from build123d import *

# Parameters (mm, degrees)
SKETCH1_R           = 1.65
BOSS_EXTRUDE1_DEPTH = 3
BOSS_EXTRUDE2_START = -3
BOSS_EXTRUDE2_DEPTH = 3
SKETCH3_R           = 1.35
CUT_EXTRUDE1_DEPTH  = 3
BOSS_EXTRUDE3_START = 2
SKETCH4_R           = 2.85
SKETCH4_R_2         = 1.35
BOSS_EXTRUDE3_DEPTH = 2


with BuildPart() as part:
    # Sketch1 → Boss-Extrude1 (new body)
    with BuildSketch(Plane(origin=(0, 0, 0), x_dir=(1, 0, 0), z_dir=(0, 1, 0))):
        with BuildLine():
            Line((-91, 63), (-11.779218989, 63))
            ThreePointArc((-11.779218989, 63), (-9.093788212, 62.217636961), (-7.248750147, 60.115384615))
            ThreePointArc((-7.248750147, 60.115384615), (0, 55.5), (7.248750147, 60.115384615))
            ThreePointArc((7.248750147, 60.115384615), (9.093788212, 62.217636961), (11.779218989, 63))
            Line((11.779218989, 63), (91, 63))
            ThreePointArc((91, 63), (94.535533906, 61.535533906), (96, 58))
            Line((96, 58), (96, -58))
            ThreePointArc((96, -58), (94.535533906, -61.535533906), (91, -63))
            Line((91, -63), (11.779218989, -63))
            ThreePointArc((11.779218989, -63), (9.093788212, -62.217636961), (7.248750147, -60.115384615))
            ThreePointArc((7.248750147, -60.115384615), (0, -55.5), (-7.248750147, -60.115384615))
            ThreePointArc((-7.248750147, -60.115384615), (-9.093788212, -62.217636961), (-11.779218989, -63))
            Line((-11.779218989, -63), (-91, -63))
            ThreePointArc((-91, -63), (-94.535533906, -61.535533906), (-96, -58))
            Line((-96, -58), (-96, 58))
            ThreePointArc((-96, 58), (-94.535533906, 61.535533906), (-91, 63))
        make_face()
        with Locations(Location((-91, 58, 0), (0, 0, 270))):
            Circle(SKETCH1_R, mode=Mode.SUBTRACT)
        with Locations(Location((91, 58, 0), (0, 0, 270))):
            Circle(SKETCH1_R, mode=Mode.SUBTRACT)
        with Locations(Location((91, -58, 0), (0, 0, 270))):
            Circle(SKETCH1_R, mode=Mode.SUBTRACT)
        with Locations(Location((-91, -58, 0), (0, 0, 270))):
            Circle(SKETCH1_R, mode=Mode.SUBTRACT)
        with BuildLine():
            Line((-81, 53), (-15, 53))
            ThreePointArc((-15, 53), (-7.928932188, 50.071067812), (-5, 43))
            Line((-5, 43), (-5, -43))
            ThreePointArc((-5, -43), (-7.928932188, -50.071067812), (-15, -53))
            Line((-15, -53), (-81, -53))
            ThreePointArc((-81, -53), (-84.535533906, -51.535533906), (-86, -48))
            Line((-86, -48), (-86, 48))
            ThreePointArc((-86, 48), (-84.535533906, 51.535533906), (-81, 53))
        make_face(mode=Mode.SUBTRACT)
        with BuildLine():
            Line((86, -48), (86, 48))
            ThreePointArc((86, 48), (84.535533906, 51.535533906), (81, 53))
            Line((81, 53), (15, 53))
            ThreePointArc((15, 53), (7.928932188, 50.071067812), (5, 43))
            Line((5, 43), (5, -43))
            ThreePointArc((5, -43), (7.928932188, -50.071067812), (15, -53))
            Line((15, -53), (81, -53))
            ThreePointArc((81, -53), (84.535533906, -51.535533906), (86, -48))
        make_face(mode=Mode.SUBTRACT)
    extrude(amount=BOSS_EXTRUDE1_DEPTH)

    # Sketch2 → Boss-Extrude2 (add)
    with BuildSketch(Plane(origin=(0, 3, 0), x_dir=(1, 0, 0), z_dir=(0, 1, 0)).offset(BOSS_EXTRUDE2_START)):
        with BuildLine():
            Line((-42, -39.5), (-86, -39.5))
            Line((-86, -39.5), (-86, -48))
            ThreePointArc((-86, -48), (-85.942088629, -48.758788496), (-85.769696007, -49.5))
            Line((-85.769696007, -49.5), (-42, -49.5))
            Line((-42, -49.5), (-7.400657923, -49.5))
            ThreePointArc((-7.400657923, -49.5), (-5.619343819, -46.464576398), (-5, -43))
            Line((-5, -43), (-5, -39.5))
            Line((-5, -39.5), (-42, -39.5))
        make_face()
        Polygon((-86, 18.5), (-86, 8.5), (-42, 8.5), (-5, 8.5), (-5, 18.5), (-42, 18.5), align=None)
    extrude(amount=BOSS_EXTRUDE2_DEPTH)

    # Sketch3 → Cut-Extrude1 (cut)
    with BuildSketch(Plane(origin=(0, 3, 0), x_dir=(1, 0, 0), z_dir=(0, 1, 0))):
        with Locations(Location((-42, -44.5, 0), (0, 0, 270))):
            Circle(SKETCH3_R)
        with Locations(Location((-91, -44.5, 0), (0, 0, 270))):
            Circle(SKETCH3_R)
        with Locations(Location((-42, 13.5, 0), (0, 0, 270))):
            Circle(SKETCH3_R)
        with Locations(Location((-91, 13.5, 0), (0, 0, 270))):
            Circle(SKETCH3_R)
    extrude(amount=-CUT_EXTRUDE1_DEPTH, mode=Mode.SUBTRACT)

    # Sketch4 → Boss-Extrude3 (add)
    # profile 1 of 4: a face of its own
    with BuildSketch(Plane(origin=(0, 3, 0), x_dir=(1, 0, 0), z_dir=(0, 1, 0)).offset(BOSS_EXTRUDE3_START)):
        with Locations(Location((-91, 13.5, 0), (0, 0, 90))):
            Circle(SKETCH4_R)
        with Locations(Location((-91, 13.5, 0), (0, 0, 270))):
            Circle(SKETCH4_R_2, mode=Mode.SUBTRACT)
    # profile 2 of 4: a face of its own
    with BuildSketch(Plane(origin=(0, 3, 0), x_dir=(1, 0, 0), z_dir=(0, 1, 0)).offset(BOSS_EXTRUDE3_START)):
        with Locations(Location((-91, -44.5, 0), (0, 0, 90))):
            Circle(SKETCH4_R)
        with Locations(Location((-91, -44.5, 0), (0, 0, 270))):
            Circle(SKETCH4_R_2, mode=Mode.SUBTRACT)
    # profile 3 of 4: a face of its own
    with BuildSketch(Plane(origin=(0, 3, 0), x_dir=(1, 0, 0), z_dir=(0, 1, 0)).offset(BOSS_EXTRUDE3_START)):
        with Locations(Location((-42, -44.5, 0), (0, 0, 90))):
            Circle(SKETCH4_R)
        with Locations(Location((-42, -44.5, 0), (0, 0, 270))):
            Circle(SKETCH4_R_2, mode=Mode.SUBTRACT)
    # profile 4 of 4: a face of its own
    with BuildSketch(Plane(origin=(0, 3, 0), x_dir=(1, 0, 0), z_dir=(0, 1, 0)).offset(BOSS_EXTRUDE3_START)):
        with Locations(Location((-42, 13.5, 0), (0, 0, 90))):
            Circle(SKETCH4_R)
        with Locations(Location((-42, 13.5, 0), (0, 0, 270))):
            Circle(SKETCH4_R_2, mode=Mode.SUBTRACT)
    extrude(amount=-BOSS_EXTRUDE3_DEPTH)


solid = part.part
Could you check a few things on this model? Use its own coordinates, in mm. A direction names the side the tool comes from. Coordinates: 2 decimals unless noted, no trailing zeros. Order: outer loops, then holes, each group sorted by start corner. A loop starts at its lowest first (then second) coordinate and runs counter-clockwise, first axis right, second up. Notation, with made-up numbers: (27, -16.75) -> (40, -16.75) arc R8 ccw to (40, -3.75) -> close; hole circle Ø3 at (67.5, 36.25). An arc over 180 degrees is marked (long way). One line per item, written item: value. Start each with the question number.
1) We'd pull the mould along X, two halves only. Please class faces 1 (the flat face through (-41, 5, -15)), 2 (the cylindrical face through (95, 1, 61)), 3 (the cylindrical face through (-39.472, 4.014, 43.185)): +X half, -X half, draft (parallel to the pull), parting line (faces both ways), or undercut.
2) Imagine slicing it at D-D on x = -2. List the corners of the cut face in (y, z) for me, plus the area to 3 significant figures.
3) Imagine slicing it at A-A on y = 3.95. List the corners of the cut face in (x, z) for me.
4) I'm going to push flat-ended pins straight in: pin 1 (2 mm diameter, centred on x = 9, y = 2, fed in from +Z); pin 2 (4.5 mm diameter, centred on x = -91, z = 58, fed in from +Y); pin 3 (2 mm diameter, centred on x = -32, z = 38, fed in from -Y); pin 4 (1.5 mm diameter, centred on y = 4, z = -13.5, fed in from -X). Where does each tip first touch, or does it pass through?
5) Imagine slicing it at B-B on z = -30.5. List the corners of the cut face in (x, y) for me, plus the area to 3 significant figures.
6) If I drill on L1, parallel to Z at x = -91, y = 0.9; L2, parallel to Z at x = -38.5, y = 1.9; L3, parallel to X at y = 1.2, z = -13.5, over which ranges is the centre line in solid material (lowest first)? Write a range as [from, to].
7) Imagine slicing it at C-C on x = 62. List the corners of the cut face in (y, z) for me.
8) Which directions (+Z, -Z, +X, -X, +Y, -Y) give clear straight access to the entire face, cutting with the end or side of a thin tool? Please do faces 4 (the cylindrical face through (-93.826, 4.014, -13.129)), 5 (the cylindrical face through (8.01, 1.48, -50.15)), 6 (the flat face through (-90, 5, 43)).
Answer list:
1. face 1: draft
1. face 2: +X half
1. face 3: undercut
2. outline: (0, -55.75) -> (3, -55.75) -> (3, 55.75) -> (0, 55.75) -> close
2. area: 335 mm2
3. outline: circle Ø5.7 at (-91, -13.5); circle Ø5.7 at (-91, 44.5); circle Ø5.7 at (-42, -13.5); circle Ø5.7 at (-42, 44.5); hole circle Ø2.7 at (-91, -13.5); hole circle Ø2.7 at (-91, 44.5); hole circle Ø2.7 at (-42, -13.5); hole circle Ø2.7 at (-42, 44.5)
4. pin 1: stops at z = 62.67
4. pin 2: stops at y = 3
4. pin 3: passes through
4. pin 4: stops at x = -93.85
5. outline: (-96, 0) -> (-86, 0) -> (-86, 3) -> (-96, 3) -> close; (-5, 0) -> (5, 0) -> (5, 3) -> (-5, 3) -> close; (86, 0) -> (96, 0) -> (96, 3) -> (86, 3) -> close
5. area: 90.0 mm2
6. L1: z = [-63, -59.65], [-56.35, -14.85], [-12.15, 43.15], [45.85, 56.35], [59.65, 63]
6. L2: z = [-63, -53], [-18.5, -8.5], [39.5, 49.5], [53, 63]
6. L3: x = [-96, -92.35], [-89.65, -43.35], [-40.65, 5], [86, 96]
7. outline: (0, -63) -> (3, -63) -> (3, -53) -> (0, -53) -> close; (0, 53) -> (3, 53) -> (3, 63) -> (0, 63) -> close
8. face 4: +Y
8. face 5: +Y, -Y
8. face 6: +Z, -Z, +X, -X, +Y
